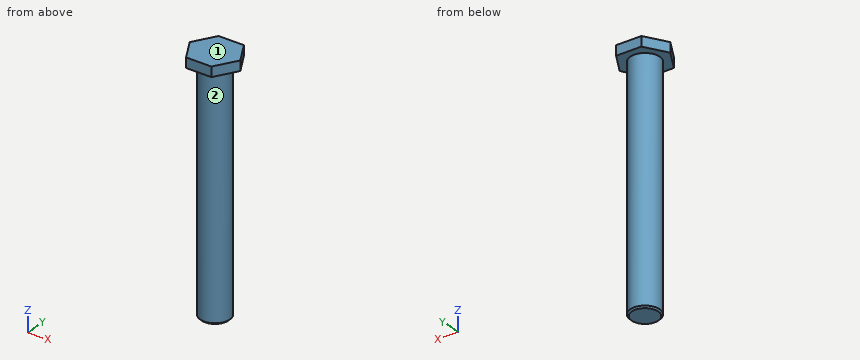
Autodesk Inventor part; units mm, degrees
ref_plane "YZ Plane" through (0, 0, 0) normal (1, 0, 0) x (0, 1, 0)
ref_plane "XZ Plane" through (0, 0, 0) normal (0, 1, 0) x (-1, 0, 0)
ref_plane "XY Plane" through (0, 0, 0) normal (0, 0, 1) x (1, 0, 0)
sketch "Sketch1" plane through (0, 0, 0) normal (0, 0, 1) x (1, 0, 0)
  circle A0 centre (-414.4261, -56.251) radius 4.7625
  point P0 (0, 0)
  dimension "d0" = 9.525
extrude "Extrusion1" add sketch "Sketch1" against normal blind 76.2
sketch "Sketch2" plane through (-414.4261, -56.251, 0) normal (0, 0, 1) x (1, 0, 0)
  circle A0 centre (0, 0) radius 4.7625
  line L0 (-8.2489, 0) -> (-4.1244, 7.1437)
  line L1 (-4.1244, 7.1437) -> (4.1244, 7.1438)
  line L2 (4.1244, 7.1438) -> (8.2489, 0)
  line L3 (8.2489, 0) -> (4.1244, -7.1437)
  line L4 (4.1244, -7.1437) -> (-4.1244, -7.1438)
  line L5 (-4.1244, -7.1438) -> (-8.2489, 0)
  point P0 (414.4261, 56.251)
  dimension "d3" = 14.2875
extrude "Extrusion2" add sketch "Sketch2" along normal blind 3.175 contours A0 | L0 L1 L2 L3 L4 L5
thread "Thread1"
chamfer "Chamfer1" distance 0.508 angle 45 1 edges at (-419.1886, -56.251, -76.2)
properties part number "375 bolt x4" material "Steel"
Source: CAD feature listing. Evaluate the final solid. Frame: model axes, mm. Face numbers are marked on the shaded views. A direction names the side the tool comes from. Round coordinates to 2 decimals unless told otherwise and drop trailing zeros. Loops run counter-clockwise (first coordinate to the right, second up) from the corner with the lowest first, then second, coordinate; pieces in that order, holes last. Notation, with made-up numbers: (-11, 74) -> (15, 74) arc R28 cw to (15, 102) -> close; hole circle Ø2 at (-8, 27). An arc over 180 degrees is marked (long way). Answer as a JSON object with one key per item and string values. Group by question number.
Q1. Section query C-C (y = -62). Output: boundary loops of the cut face in (x, z) (3 decimals), plus the area to 3 significant figures.
Q2. Ray query, line 1 (Z direction, x = -420, y = -57.25) (3 decimals); line 2 (Y direction, x = -414.75, z = -37); line 3 (X direction, y = -54, z = -25). Return the intervals inside material, ascending. Write a range as from..to.
Q3. Access query for the marked faces 1 and 2. Directions: +Z, -Z, +X, -X, +Y, -Y. A direction counts if a zero-diameter tool reaches every point of the face in a straight line with its end or side. Return the directions, or none.
Q4. Contact query for flat-ended pins moving along their axis: P1, Ø8, axis at x = -411, z = -28, coming from the -Y side; P2, Ø5, axis at x = -413.5, z = -35.5, coming from the +Y side; P3, Ø5, axis at x = -409.5, z = -10, coming from the +Y side. Output: stop coordinate, or through.
Q5. Section query A-A (z = -19). Output: boundary loops of the cut face in (x, y) (1 decimal), plus the area to 3 significant figures.
Q6. Section query B-B (x = -421.25). Output: boundary loops of the cut face in (y, z) (3 decimals).
Completed:
{
 "1": {"outline": "(-419.356, 0) -> (-409.496, 0) -> (-409.496, 3.175) -> (-419.356, 3.175) -> close", "area": "31.3 mm²"},
 "2": {"line 1": "0..3.175", "line 2": "-61..-51.5", "line 3": "-418.62..-410.23"},
 "3": {"face 1": "+Z, +X, -X, +Y, -Y", "face 2": "-Z"},
 "4": {"P1": "y = -61.01", "P2": "y = -51.49", "P3": "y = -52.15"},
 "5": {"outline": "circle Ø9.5 at (-414.4, -56.3)", "area": "71.3 mm²"},
 "6": {"outline": "(-58.719, 0) -> (-53.783, 0) -> (-53.783, 3.175) -> (-58.719, 3.175) -> close"}
}
